Design review of the part built by this model. Coordinates are the model's own, in mm. A direction names the side the tool comes from. Coordinates: 2 decimals unless noted, no trailing zeros. Loops run counter-clockwise (first coordinate to the right, second up) from the corner with the lowest first, then second, coordinate; pieces in that order, holes last. Notation, with made-up numbers: M -16.5,61.5 L -2.5,61.5 A24 ccw -2.5,87.5 Z; hole C 33.25,47 d7. An arc over 180 degrees is marked long. Answer as a JSON object with one key per item and string values. Group by question number.
1. Consider section C-C (x = 15). State the section outline as (y, z) points, then the cut area to 3 significant figures.
2. To check wall thickness, follow probe 1 along X at (y, z) = (-40, -0.25); probe 2 along Z at (x, y) = (0, -39); probe 3 along Z at (x, y) = (22, 0). State the ranges of each line that lie inside material, in increasing order.
3. Machinability: for faces 4 (the flat face through (-20, -37, 0)), 5 (the flat face through (-20, 0, 0)), 6 (the flat face through (20, 0, 0)), which of the approach directions +Z, -Z, +X, -X, +Y, -Y give a long, thin tool a straight path to every point of the face, cutting with its end or side? Answer none if there is none.
4. Consider section A-A (y = 31). State the section outline as (x, z) points, then the cut area to 3 significant figures.
5. Consider section B-B (x = -25.5). State the section outline as (y, z) points.
6. Consider section D-D (y = -31). State the section outline as (x, z) points, then the cut area to 3 significant figures.
7. Draft analysis for pull direction X (two halves, no side actions). For faces 1 (the cylindrical face through (-13.62, 41.06, 0.51)), 2 (the flat face through (0, 1, 3.1)), 3 (the flat face through (24.93, 27.74, 0.04)), state which applies: +X half, -X half, draft (parallel to the pull), parting line (faces both ways), or undercut.
8. Insertion check: pin 1 (7 mm diameter, centred on x = 15.24, y = 31, fed in from +Z); pin 2 (3 mm diameter, centred on x = -20, z = 0, fed in from -Y); pin 3 (1 mm diameter, centred on x = 12, z = 0.5, fed in from +Y); pin 4 (2 mm diameter, centred on y = 0, z = 0, fed in from +X). Each pin has a flat end and moves straight along its axis. Give the tip position at first contact, or say it passes through.
from build123d import *

# Parameters (mm, degrees)
EXTRUDE_1_4_DEPTH = 3.1
SKETCH4_R         = 1.7
M4_DRILL_DEPTH    = 8
SKETCH5_R         = 1.7
M4_DRILL2_DEPTH   = 8
SKETCH6_R         = 2.2
M4_THROUGH_DEPTH  = 6.2
SKETCH7_R         = 1.3
M3_DRILL_DEPTH    = 10


with BuildPart() as part:
    # Sketch1 → 1/4 (new, symmetric)
    with BuildSketch(Plane.XY):
        Polygon((-20, 45), (20, 45), (30, 10), (30, -45), (-30, -45), (-30, 10), align=None)
    extrude(amount=EXTRUDE_1_4_DEPTH, both=True)

    # Sketch4 → M4_DRILL (cut)
    with BuildSketch(Plane(origin=(0, 45, 0), x_dir=(1, 0, 0), z_dir=(0, 1, 0))):
        with Locations(Location((-12, 0, 0), (0, 0, 180))):
            Circle(SKETCH4_R)
        with Locations((12, 0)):
            Circle(SKETCH4_R)
    extrude(amount=-M4_DRILL_DEPTH, mode=Mode.SUBTRACT)

    # Sketch5 → M4_DRILL2 (cut)
    with BuildSketch(Plane(origin=(0, -45, 0), x_dir=(-1, 0, 0), z_dir=(0, -1, 0))):
        with Locations(Location((-20, 0, 0), (0, 0, 180))):
            Circle(SKETCH5_R)
        with Locations((20, 0)):
            Circle(SKETCH5_R)
        with Locations(Location((0, 0, 0), (0, 0, 180))):
            Circle(SKETCH5_R)
    extrude(amount=-M4_DRILL2_DEPTH, mode=Mode.SUBTRACT)

    # Sketch6 → M4_through (cut)
    with BuildSketch(Plane.XY.offset(3.1)):
        with Locations((-25.2375, -31)):
            Circle(SKETCH6_R)
        with Locations((25.2375, -31)):
            Circle(SKETCH6_R)
        with Locations((-15.2375, 31)):
            Circle(SKETCH6_R)
        with Locations((15.2375, 31)):
            Circle(SKETCH6_R)
    extrude(amount=-M4_THROUGH_DEPTH, mode=Mode.SUBTRACT)

    # Sketch7 → M3_Drill (cut)
    with BuildSketch(Plane.ZY.offset(30)):
        with Locations(Location((0, 0, 0), (0, 0, 270))):
            Circle(SKETCH7_R)
    m3_drill = extrude(amount=-M3_DRILL_DEPTH, mode=Mode.SUBTRACT)

    # Mirror1: M3_Drill across plane
    add(m3_drill.mirror(Plane(origin=(0, 0, 0), x_dir=(0, 0, 1), z_dir=(1, 0, 0))), mode=Mode.SUBTRACT)


solid = part.part
Findings below:
{
 "1": {"outline": "M -45,-3.1 L 28.81,-3.1 L 28.81,3.1 L -45,3.1 Z; M 33.19,-3.1 L 45,-3.1 L 45,3.1 L 33.19,3.1 Z", "area": "531 mm^2"},
 "2": {"probe 1": "x = -30 to -21.68, -18.32 to -1.68, 1.68 to 18.32, 21.68 to 30", "probe 2": "z = -3.1 to -1.7, 1.7 to 3.1", "probe 3": "z = -3.1 to -1.3, 1.3 to 3.1"},
 "3": {"face 4": "-Y", "face 5": "-X", "face 6": "+X"},
 "4": {"outline": "M -24,-3.1 L -17.44,-3.1 L -17.44,3.1 L -24,3.1 Z; M -13.04,-3.1 L 13.04,-3.1 L 13.04,3.1 L -13.04,3.1 Z; M 17.44,-3.1 L 24,-3.1 L 24,3.1 L 17.44,3.1 Z", "area": "243 mm^2"},
 "5": {"outline": "M -45,-3.1 L -33.18,-3.1 L -33.18,3.1 L -45,3.1 Z; M -28.82,-3.1 L 25.75,-3.1 L 25.75,3.1 L -28.82,3.1 Z; hole C 0,0 d2.6"},
 "6": {"outline": "M -30,-3.1 L -27.44,-3.1 L -27.44,3.1 L -30,3.1 Z; M -23.04,-3.1 L 23.04,-3.1 L 23.04,3.1 L -23.04,3.1 Z; M 27.44,-3.1 L 30,-3.1 L 30,3.1 L 27.44,3.1 Z", "area": "317 mm^2"},
 "7": {"face 1": "undercut", "face 2": "draft", "face 3": "+X half"},
 "8": {"pin 1": "stops at z = 3.1", "pin 2": "stops at y = -37", "pin 3": "stops at y = 37", "pin 4": "stops at x = 20"}
}
